Autodesk Inventor part; units mm, degrees
ref_plane "YZ Plane" through (0, 0, 0) normal (1, 0, 0) x (0, 1, 0)
ref_plane "XZ Plane" through (0, 0, 0) normal (0, 1, 0) x (-1, 0, 0)
ref_plane "XY Plane" through (0, 0, 0) normal (0, 0, 1) x (1, 0, 0)
sketch "Sketch1" plane through (0, 0, 0) normal (0, 0, 1) x (1, 0, 0)
  line L0 (-16.6819, 17.4202) -> (21.4181, 17.4202)
  line L1 (21.4181, 17.4202) -> (21.4181, -71.4798)
  line L2 (21.4181, -71.4798) -> (-16.6819, -71.4798)
  line L3 (-16.6819, -71.4798) -> (-16.6819, 17.4202)
  point P0 (0, 0)
  dimension "d0" = 38.1
  dimension "d1" = 88.9
extrude "Extrusion1" add sketch "Sketch1" along normal blind 254
sketch "Sketch2" plane through (21.4181, -71.4798, 0) normal (1, 0, 0) x (0, 0, -1)
  line L0 (0, 0) -> (-254, 0)
  arc A0 (-76.2, 0) -> (-177.8, 0) centre (-127, -116.3974) ccw
  point P0 (0, 71.4798)
  dimension "d4" = 127
  dimension "d5" = 76.2
  dimension "d6" = 76.2
extrude "Extrusion2" cut sketch "Sketch2" against normal blind 76.2
equation "\"d6\" = d5"
properties part number "RailMount2x4_NERDS"
The listing builds one solid part. Answer for the finished solid, in the listing's coordinates (mm). Round coordinates to 2 decimals unless told otherwise and drop trailing zeros. Loops run counter-clockwise (first coordinate to the right, second up) from the corner with the lowest first, then second, coordinate; pieces in that order, holes last. Notation, with made-up numbers: (57.25, 42.25) - (83.25, 42.25) arc R27 cw to (83.25, 60.25) - close; hole circle Ø2 at (89, -9.75). An arc over 180 degrees is marked (long way). Use one line per item in the form item = value. Start each with the question number.
1. The part is cut by section B-B on z = 167.5. Determine the outline of the cut face in (x, y).
2. The part is cut by section A-A on x = -1. Determine the outline of the cut face in (y, z), then the cut area to 3 significant figures.
3. The part is cut by section C-C on z = 115. Determine the outline of the cut face in (x, y).
4. Consider line 1 (Y direction, x = -10, z = 175); line 2 (Y direction, x = -7, z = 176). Determine where each line is inside the solid, lowest interval first. Write a range as [from, to].
Geometry check:
q1.outline = (-16.68, -67.51) - (21.42, -67.51) - (21.42, 17.42) - (-16.68, 17.42) - close
q2.outline = (-71.48, 0) - (17.42, 0) - (17.42, 254) - (-71.48, 254) - (-71.48, 177.8) arc R127 cw to (-71.48, 76.2) - close
q2.area = 21,900 mm^2
q3.outline = (-16.68, -61.45) - (21.42, -61.45) - (21.42, 17.42) - (-16.68, 17.42) - close
q4.line_1 = [-70.3, 17.42]
q4.line_2 = [-70.71, 17.42]
